For this review, take the finished solid that the model builds, in its own axes (mm). A direction names the side the tool comes from. Round coordinates to 2 decimals unless told otherwise and drop trailing zeros. Loops run counter-clockwise (first coordinate to the right, second up) from the corner with the lowest first, then second, coordinate; pieces in that order, holes last.
1) Insertion check: pin 1 (10 mm diameter, centred on y = 13.5, z = 14.5, fed in from -X); pin 2 (5 mm diameter, centred on x = 13, z = 3.5, fed in from +Y); pin 3 (1 mm diameter, centred on x = 44.5, z = 12.5, fed in from -Y). Each pin has a flat end and moves straight along its axis. Give the tip position at first contact, or say it passes through.
2) Take a section at B-B (x = 16.5). State the section outline as (y, z) points.
3) Take a section at D-D (x = 5). State the section outline as (y, z) points, then the cut area to 3 significant figures.
4) Take a section at C-C (z = 12.75). State the section outline as (x, y) points, then the cut area to 3 significant figures.
5) Take a section at A-A (y = 13). State the section outline as (x, z) points.
6) Wall thickness on L1, parallel to Z at x = 5.5, y = 43.5; L2, parallel to X at y = 18, z = 7.25: over which ranges is each line inside the solid? List them lowest first.
7) Tool access review of faces 1 (the cylindrical face through (3.04, 56.14, 0.9)), 2 (the flat face through (15, 3, 10.8)), 3 (the flat face through (31, 6, 11)), 4 (the flat face through (3, 44, 17.2)): name each direction out of +Z, -Z, +X, -X, +Y, -Y from which nothing blocks a thin tool from reaching the whole face with its end or side.
8) Mouldability with a two-part tool opening along Y and no side actions: class faces 5 (the flat face through (3, 15, 10.8)), 6 (the flat face through (50, 3, 14)), 7 (the flat face through (29, 0, 14)) as pulls with the +Y half, pulls with the -Y half, needs draft (parallel to the pull), parting line crosses it, or undercut.
```python
from build123d import *

# Parameters (mm, degrees)
AUFSATZ_LINEAR_AUSTRAGEN1_DEPTH = 28
AUFSATZ_LINEAR_AUSTRAGEN2_DEPTH = 6
SKIZZE3_W                       = 6.4
SKIZZE3_H                       = 11
SKIZZE3_H_2                     = 10
SCHNITT_LINEAR_AUSTRAGEN1_DEPTH = 7
SKIZZE4_W                       = 11
SKIZZE4_H                       = 6.4
SKIZZE4_W_2                     = 10
SCHNITT_LINEAR_AUSTRAGEN2_DEPTH = 7
VERRUNDUNG1_R                   = 3


with BuildPart() as part:
    # Skizze1 → Aufsatz-Linear austragen1 (new body)
    with BuildSketch(Plane.XY):
        Polygon((0, 0), (0, 57), (6, 57), (6, 6), (57, 6), (57, 0), align=None)
    extrude(amount=AUFSATZ_LINEAR_AUSTRAGEN1_DEPTH)

    # Skizze2 → Aufsatz-Linear austragen2 (add)
    with BuildSketch(Plane.XY.offset(28)):
        Polygon((6, 57), (6, 6), (57, 6), align=None)
    extrude(amount=-AUFSATZ_LINEAR_AUSTRAGEN2_DEPTH)

    # Skizze3 → Schnitt-Linear austragen1 (cut, through all)
    with BuildSketch(Plane(origin=(6, 0, 0), x_dir=(0, 0, -1), z_dir=(1, 0, 0))):
        with Locations((-14, 44.5)):
            Rectangle(SKIZZE3_W, SKIZZE3_H)
        with Locations((-14, 15)):
            Rectangle(SKIZZE3_W, SKIZZE3_H_2)
    extrude(amount=-SCHNITT_LINEAR_AUSTRAGEN1_DEPTH, mode=Mode.SUBTRACT)

    # Skizze4 → Schnitt-Linear austragen2 (cut, through all)
    with BuildSketch(Plane(origin=(0, 6, 0), x_dir=(1, 0, 0), z_dir=(0, 1, 0))):
        with Locations((44.5, -14)):
            Rectangle(SKIZZE4_W, SKIZZE4_H)
        with Locations((15, -14)):
            Rectangle(SKIZZE4_W_2, SKIZZE4_H)
    extrude(amount=-SCHNITT_LINEAR_AUSTRAGEN2_DEPTH, mode=Mode.SUBTRACT)

    # Verrundung1
    verrundung1_edges = [part.edges().sort_by_distance(p)[0] for p in [
        (3, 57, 28),
        (3, 57, 0),
        (57, 3, 28),
        (57, 3, 0),
    ]]
    fillet(verrundung1_edges, radius=VERRUNDUNG1_R)


solid = part.part
```
Response:
1. pin 1: stops at x = 0
1. pin 2: stops at y = 6
1. pin 3: passes through
2. outline: (0, 0) - (6, 0) - (6, 10.8) - (0, 10.8) - close; (0, 17.2) - (6, 17.2) - (6, 22) - (46.5, 22) - (46.5, 28) - (0, 28) - close
3. outline: (0, 0) - (54, 0) arc R3 ccw to (57, 3) - (57, 25) arc R3 ccw to (54, 28) - (0, 28) - close; hole (10, 10.8) - (20, 10.8) - (20, 17.2) - (10, 17.2) - close; hole (39, 10.8) - (50, 10.8) - (50, 17.2) - (39, 17.2) - close
3. area: 1,460 mm2
4. outline: (0, 0) - (10, 0) - (10, 6) - (6, 6) - (6, 10) - (0, 10) - close; (0, 20) - (6, 20) - (6, 39) - (0, 39) - close; (0, 50) - (6, 50) - (6, 57) - (0, 57) - close; (20, 0) - (39, 0) - (39, 6) - (20, 6) - close; (50, 0) - (57, 0) - (57, 6) - (50, 6) - close
4. area: 396 mm2
5. outline: (0, 0) - (6, 0) - (6, 10.8) - (0, 10.8) - close; (0, 17.2) - (6, 17.2) - (6, 22) - (50, 22) - (50, 28) - (0, 28) - close
6. L1: z = 0 to 10.8, 17.2 to 28
6. L2: x = 0 to 6
7. face 1: -Z, +X, -X, +Y
7. face 2: +Y, -Y
7. face 3: -Z, +X, +Y
7. face 4: +X, -X
8. face 5: undercut
8. face 6: needs draft
8. face 7: pulls with the -Y half
